The model under review builds one solid part; all positions refer to its coordinate system, in mm. Face numbers are marked on the shaded views. A direction names the side the tool comes from. Coordinates: 2 decimals unless noted, no trailing zeros. Loops run counter-clockwise (first coordinate to the right, second up) from the corner with the lowest first, then second, coordinate; pieces in that order, holes last. Notation, with made-up numbers: (67, 14.25) - (115, 14.25) arc R17 ccw to (115, 37.25) - close; hole circle Ø7 at (21, 1). An arc over 180 degrees is marked (long way). One line per item, written item: value. Start each with the question number.
1. Insertion check: P1, Ø4, axis at x = -20, z = -7.25, coming from the +Y side; P2, Ø1.9, axis at x = -20.5, y = 4, coming from the -Z side; P3, Ø1.5, axis at x = -20, z = -22.45, coming from the +Y side; P4, Ø3, axis at x = -39, y = 6, coming from the +Z side. Each pin has a flat end and moves straight along its axis. Give the tip position at first contact, or say it passes through.
2. We need section B-B, the plane z = -3.5. Give the boundary of the cut face in (x, y), then the cut area to 3 significant figures.
3. To check wall thickness, follow line 1 (Z direction, x = -40, y = 11.25); line 2 (Z direction, x = -8.1, y = 5); line 3 (X direction, y = 10.35, z = -22.45). State the ranges of each line that lie inside material, in increasing order.
4. We need section A-A, the plane x = -3.5. Give the boundary of the cut face in (y, z).
5. We need section C-C, the plane y = 1.25. Give the boundary of the cut face in (x, z).
6. We need section D-D, the plane z = -20. Give the boundary of the cut face in (x, y), then the cut area to 3 significant figures.
7. Mouldability with a two-part tool opening along Y and no side actions: class the marked faces 1, 2, 3 and 4 as +Y half, -Y half, draft (parallel to the pull), parting line (faces both ways), or undercut.
8. For the marked faces 5, 6 and 7, list the 3-axis set-ups (+Z, -Z, +X, -X, +Y, -Y) from which the entire face can be reached by the end or side of a thin tool; tool diameter is ignored.
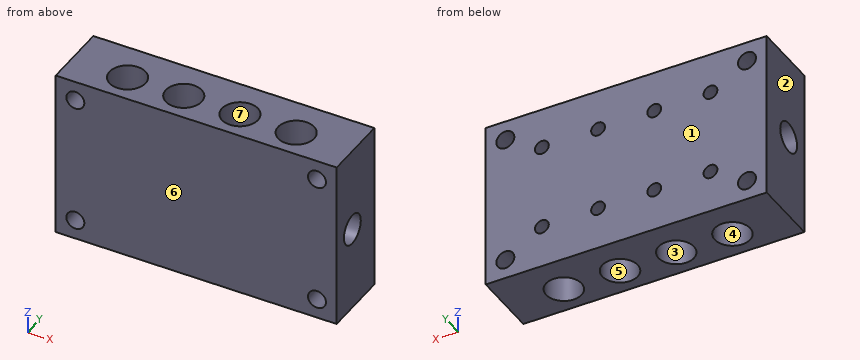
Autodesk Inventor part; units mm, degrees
ref_plane "Work Plane1" through (0, 0, -15) normal (0, 0, 1) x (1, 0, 0)
ref_plane "Work Plane2" through (0, 5, -14.6) normal (0, 0, 1) x (1, 0, 0)
ref_plane "Work Plane3" through (0, 6, -30) normal (0, -1, 0) x (1, 0, 0)
sketch "Sketch1" plane through (0, 0, 0) normal (1, 0, 0) x (0, 1, 0)
  line L0 (0, 0) -> (12, 0)
  line L1 (12, 0) -> (12, -30)
  line L2 (12, -30) -> (0, -30)
  line L3 (0, -30) -> (0, 0)
  circle A0 centre (5, -15) radius 0.4
  dimension "d0" = 30
  dimension "d1" = 12
  dimension "d2" = 5
  dimension "d3" = 15
  dimension "d4" = 0.8
extrude "Extrusion1" add sketch "Sketch1" against normal blind 50
ref_plane "Work Plane1" through (0, 0, -15) normal (0, 0, 1) x (1, 0, 0)
sketch "Sketch2" plane through (0, 0, 0) normal (0, 0, 1) x (1, 0, 0)
  line L0 (0, 0) -> (-50, 0)
  line L1 (0, 0) -> (0, 12)
  circle A0 centre (-10, 5) radius 3.2
  dimension "d7" = 6.4
  dimension "d8" = 5
  dimension "d9" = 10
extrude "Extrusion4" cut sketch "Sketch2" against normal blind 10.8
pattern_linear "Rectangular Pattern1" count 4 spacing 10 along (-1, 0, 0) of "Extrusion4"
ref_plane "Work Plane2" through (0, 5, -14.6) normal (0, 0, 1) x (1, 0, 0)
sketch "Sketch3" plane through (-10, 5, -10.8) normal (0, 0, 1) x (1, 0, 0)
  circle A0 centre (0, 0) radius 0.4
  circle A1 centre (0, 0) radius 3.2
  point P0 (10, -5)
  dimension "d20" = 0.8
extrude "Extrusion5" cut sketch "Sketch3" against normal blind 10 contours A0
pattern_linear "Rectangular Pattern2" count 4 spacing 10 along (-1, 0, 0) of "Extrusion5"
ref_plane "Work Plane3" through (0, 6, -30) normal (0, -1, 0) x (1, 0, 0)
sketch "Sketch4" plane through (0, 12, 0) normal (0, 1, 0) x (1, 0, 0)
  line L0 (0, 0) -> (0, 30)
  line L1 (0, 0) -> (-50, 0)
  circle A0 centre (-10, 7.25) radius 0.4
  circle A1 centre (-3.5, 3.5) radius 1.6
  dimension "d26" = 0.8
  dimension "d27" = 7.25
  dimension "d28" = 10
  dimension "d93" = 3.2
  dimension "d94" = 3.5
  dimension "d95" = 3.5
hole "Hole1" at (-10, 12, -7.25) direction (0, -1, 0) diameter 2.46 depth 7
pattern_linear "Rectangular Pattern4" count 4 spacing 10 along (-1, 0, 0) count 2 spacing 15.2 along (0, 0, -1) of "Hole1"
sketch "Sketch5" plane through (0, 0, -30) normal (0, 0, -1) x (-1, 0, 0)
  circle A0 centre (10, 5) radius 3.2
  line L0 (0, 12) -> (50, 12)
  line L1 (0, 12) -> (0, 0)
  line L2 (0, 0) -> (50, 0)
  dimension "d47" = 6.4
  dimension "d49" = 10
  dimension "d109" = 5
hole "Hole2" at (-10, 5, -30) direction (0, 0, 1) diameter 6.3 depth 10.8
pattern_linear "Rectangular Pattern5" count 4 spacing 10 along (-1, 0, 0) of "Hole2", "Extrusion4"
hole "Hole3" at (0, 5, -15) direction (-1, 0, 0) diameter 5.36 depth 7
sketch "Sketch6" plane through (-50, 0, 0) normal (-1, 0, 0) x (0, 0, 1)
  circle A0 centre (-15, 5) radius 2.15
  line L0 (-30, 0) -> (0, 0)
  dimension "d67" = 15
  dimension "d68" = 5
  dimension "d69" = 4.3
hole "Hole4" at (-50, 5, -15) direction (1, 0, 0) diameter 5.36 depth 7
hole "Hole5" at (-3.5, 12, -3.5) direction (0, -1, 0) diameter 3.2 end through all
pattern_linear "Rectangular Pattern6" count 2 spacing 43 along (-1, 0, 0) count 2 spacing 23 along (0, 0, -1) of "Hole5"
equation "\"d3\" = 0.5 * d0"
properties part number "Manifold_v5"
Findings below:
1. P1: y = 12
1. P2: z = -19.2
1. P3: y = 1.94
1. P4: z = -10.8
2. outline: (-50, 0) - (-48.1, 0) - (-48.1, 12) - (-50, 12) - close; (-44.9, 0) - (-5.1, 0) - (-5.1, 12) - (-44.9, 12) - close; (-1.9, 0) - (0, 0) - (0, 12) - (-1.9, 12) - close; hole circle Ø6.4 at (-40, 5); hole circle Ø6.4 at (-30, 5); hole circle Ø6.4 at (-20, 5); hole circle Ø6.4 at (-10, 5)
2. area: 395 mm2
3. line 1: -30 to -23.68, -21.22 to -8.48, -6.02 to 0
3. line 2: -19.2 to -15.4, -14.6 to -10.8
3. line 3: -50 to -41.23, -38.77 to -31.23, -28.77 to -21.23, -18.77 to -11.23, -8.77 to 0
4. outline: (0, -30) - (12, -30) - (12, -28.1) - (0, -28.1) - close; (0, -24.9) - (12, -24.9) - (12, -5.1) - (0, -5.1) - close; (0, -1.9) - (12, -1.9) - (12, 0) - (0, 0) - close; hole circle Ø5.36 at (5, -15)
5. outline: (-50, -30) - (0, -30) - (0, 0) - (-50, 0) - close; hole circle Ø3.2 at (-46.5, -26.5); hole circle Ø3.2 at (-46.5, -3.5); hole circle Ø3.2 at (-3.5, -26.5); hole circle Ø3.2 at (-3.5, -3.5)
6. outline: (-50, 0) - (0, 0) - (0, 12) - (-50, 12) - close; hole circle Ø6.3 at (-40, 5); hole circle Ø6.3 at (-30, 5); hole circle Ø6.3 at (-20, 5); hole circle Ø6.3 at (-10, 5)
6. area: 475 mm2
7. face 1: +Y half
7. face 2: draft
7. face 3: undercut
7. face 4: undercut
8. face 5: -Z
8. face 6: +Z, -Z, +X, -X, -Y
8. face 7: +Z
